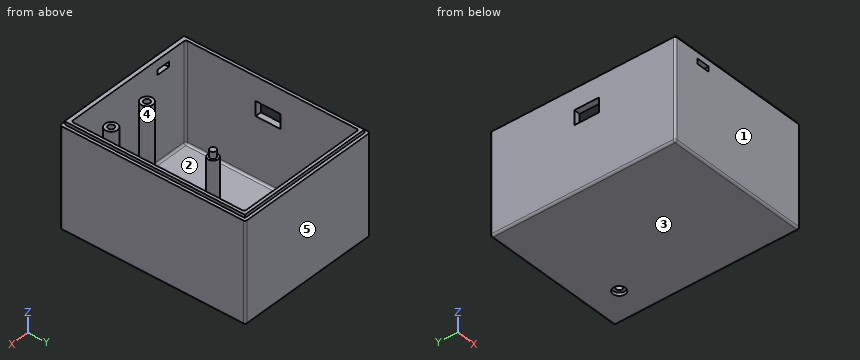
```python
from build123d import *

# Parameters (mm, degrees)
SKETCH1_W                    = 71
SKETCH1_H                    = 90
BOSS_EXTRUDE1_DEPTH          = 50
SHELL1_T                     = -3
SHELL1_THICKNESS_2_FACE_W    = 65
SHELL1_THICKNESS_2_FACE_H    = 84
SHELL1_THICKNESS_2_DEPTH     = 1
SKETCH3_W                    = 6.5
SKETCH3_H                    = 2.5
CUT_EXTRUDE1_DEPTH           = 3
SKETCH4_W                    = 7
SKETCH4_H                    = 12
CUT_EXTRUDE2_DEPTH           = 3
SKETCH5_R                    = 3
SKETCH5_R_2                  = 2.5
BOSS_EXTRUDE2_DEPTH          = 38
F_3_0_3_DIAMETER_HOLE1_D     = 3
F_3_0_3_DIAMETER_HOLE1_DEPTH = 8.5
F_3_0_3_DIAMETER_HOLE1_TIP   = 0.901290929
FILLET1_R                    = 1
FILLET2_R                    = 1
SKETCH22_R                   = 1.5
BOSS_EXTRUDE4_DEPTH          = 3.3
SKETCH23_R                   = 3
BOSS_EXTRUDE5_DEPTH          = 4
CUT_EXTRUDE3_START           = -1.5
CUT_EXTRUDE3_DEPTH           = 1.5
CUT_EXTRUDE4_DEPTH           = 68
SKETCH29_R                   = 3
CUT_EXTRUDE5_DEPTH           = 1.5
SKETCH30_R                   = 1.5
CUT_EXTRUDE6_DEPTH           = 2.5


# Read off the part's stored shape, not the designer's step: Cut-Extrude3
with BuildPart() as part:
    # Sketch1 → Boss-Extrude1 (new body)
    with BuildSketch(Plane.XY):
        Rectangle(SKETCH1_W, SKETCH1_H)
    extrude(amount=-BOSS_EXTRUDE1_DEPTH)

    # Shell1
    shell1_openings = [part.faces().sort_by_distance(p)[0] for p in [
        (0, 0, 0),
    ]]
    offset(amount=SHELL1_T, openings=shell1_openings, kind=Kind.INTERSECTION)

    # Shell1 thickness 2 face (on inner face of the shell) → Shell1 thickness 2 (cut)
    with BuildSketch(Plane(origin=(0, 0, -47), x_dir=(-1, 0, 0), z_dir=(0, 0, -1))):
        Rectangle(SHELL1_THICKNESS_2_FACE_W, SHELL1_THICKNESS_2_FACE_H)
    extrude(amount=SHELL1_THICKNESS_2_DEPTH, mode=Mode.SUBTRACT)

    # Sketch3 → Cut-Extrude1 (cut)
    with BuildSketch(Plane.XZ.offset(45)):
        with Locations((-19.75, -5.75)):
            Rectangle(SKETCH3_W, SKETCH3_H)
    extrude(amount=-CUT_EXTRUDE1_DEPTH, mode=Mode.SUBTRACT)

    # Sketch4 → Cut-Extrude2 (cut)
    with BuildSketch(Plane.ZY.offset(35.5)):
        with Locations((-15, -2)):
            Rectangle(SKETCH4_W, SKETCH4_H)
    extrude(amount=-CUT_EXTRUDE2_DEPTH, mode=Mode.SUBTRACT)

    # Sketch5 → Boss-Extrude2 (add)
    with BuildSketch(Plane.XY.offset(-48)):
        with Locations((-4.82, -37.13)):
            Circle(SKETCH5_R)
        with Locations((15.5, -37.13)):
            Circle(SKETCH5_R)
        with Locations((4.83, 3.15)):
            Circle(SKETCH5_R_2)
    extrude(amount=BOSS_EXTRUDE2_DEPTH)

    # Ø3.0 (3) Diameter Hole1
    with Locations(Plane.XY.offset(-10)):
        with Locations((-4.82, -37.13), (15.5, -37.13), (15.5, 6.05), (-4.82, 6.05)):
            Hole(F_3_0_3_DIAMETER_HOLE1_D / 2, depth=F_3_0_3_DIAMETER_HOLE1_DEPTH)
            with Locations((0, 0, -(F_3_0_3_DIAMETER_HOLE1_DEPTH + F_3_0_3_DIAMETER_HOLE1_TIP / 2))):  # 118° drill point
                Cone(0, F_3_0_3_DIAMETER_HOLE1_D / 2, F_3_0_3_DIAMETER_HOLE1_TIP, mode=Mode.SUBTRACT)

    # Fillet1
    fillet1_edges = [part.edges().sort_by_distance(p)[0] for p in [
        (-35.5, 0, -50),
        (0, -45, -50),
        (32.5, 42, -24),
        (32.5, -42, -24),
        (-32.5, -42, -24),
        (-32.5, 42, -24),
        (35.5, 0, -50),
        (0, 45, -50),
        (35.5, -45, -25),
        (-35.5, -45, -25),
        (-35.5, 45, -25),
        (35.5, 45, -25),
    ]]
    fillet(fillet1_edges, radius=FILLET1_R)

    # Fillet2
    # the kernel refuses this fillet: 1 mm, written as the material it adds along each edge
    with BuildSketch(Plane(origin=(-4.82, -37.13, -48), x_dir=(1, 0, 0), z_dir=(0, -1, 0))) as fillet2_piece_1:
        with BuildLine():
            CenterArc((3 + FILLET2_R, FILLET2_R), FILLET2_R, 180, 90)
            Line((3, FILLET2_R), (3, 0))
            Line((3, 0), (3 + FILLET2_R, 0))
        make_face()
    revolve(axis=Axis((-4.82, -37.13, -48), (0, 0, 1)))
    with BuildSketch(Plane(origin=(15.5, -37.13, -48), x_dir=(1, 0, 0), z_dir=(0, -1, 0))) as fillet2_piece_2:
        with BuildLine():
            CenterArc((3 + FILLET2_R, FILLET2_R), FILLET2_R, 180, 90)
            Line((3, FILLET2_R), (3, 0))
            Line((3, 0), (3 + FILLET2_R, 0))
        make_face()
    revolve(axis=Axis((15.5, -37.13, -48), (0, 0, 1)))
    with BuildSketch(Plane(origin=(4.83, 3.15, -48), x_dir=(1, 0, 0), z_dir=(0, -1, 0))) as fillet2_piece_3:
        with BuildLine():
            CenterArc((2.5 + FILLET2_R, FILLET2_R), FILLET2_R, 180, 90)
            Line((2.5, FILLET2_R), (2.5, 0))
            Line((2.5, 0), (2.5 + FILLET2_R, 0))
        make_face()
    revolve(axis=Axis((4.83, 3.15, -48), (0, 0, 1)))
    with BuildSketch(Plane(origin=(31.5, 42, -48), x_dir=(0, 0, 1), z_dir=(-1, 0, 0)), Plane(origin=(-31.5, -42, -48), x_dir=(0, 0, 1), z_dir=(1, 0, 0))) as fillet2_piece_4:
        with BuildLine():
            CenterArc((FILLET2_R, -FILLET2_R), FILLET2_R, 90, 90)
            Line((0, -FILLET2_R), (0, 0))
            Line((0, 0), (FILLET2_R, 0))
        make_face()
    extrude(amount=63)
    with BuildSketch(Plane(origin=(32.5, -41, -48), x_dir=(0, 0, 1), z_dir=(0, 1, 0)), Plane(origin=(-32.5, 41, -48), x_dir=(0, 0, 1), z_dir=(0, -1, 0))) as fillet2_piece_5:
        with BuildLine():
            CenterArc((FILLET2_R, -FILLET2_R), FILLET2_R, 90, 90)
            Line((0, -FILLET2_R), (0, 0))
            Line((0, 0), (FILLET2_R, 0))
        make_face()
    extrude(amount=82)
    with BuildSketch(Plane(origin=(-31.5, -41, -48), x_dir=(-1, 0, 0), z_dir=(0, 1, 0))) as fillet2_piece_6:
        with BuildLine():
            CenterArc((1 - FILLET2_R, FILLET2_R), FILLET2_R, 270, 90)
            Line((1 - FILLET2_R, 0), (1, 0))
            Line((1, 0), (1, FILLET2_R))
        make_face()
    revolve(axis=Axis((-31.5, -41, -48), (0, 0, 1)), revolution_arc=90)
    with BuildSketch(Plane(origin=(-31.5, 41, -48), x_dir=(0, 1, 0), z_dir=(1, 0, 0))) as fillet2_piece_7:
        with BuildLine():
            CenterArc((1 - FILLET2_R, FILLET2_R), FILLET2_R, 270, 90)
            Line((1 - FILLET2_R, 0), (1, 0))
            Line((1, 0), (1, FILLET2_R))
        make_face()
    revolve(axis=Axis((-31.5, 41, -48), (0, 0, 1)), revolution_arc=90)
    with BuildSketch(Plane(origin=(31.5, -41, -48), x_dir=(0, -1, 0), z_dir=(-1, 0, 0))) as fillet2_piece_8:
        with BuildLine():
            CenterArc((1 - FILLET2_R, FILLET2_R), FILLET2_R, 270, 90)
            Line((1 - FILLET2_R, 0), (1, 0))
            Line((1, 0), (1, FILLET2_R))
        make_face()
    revolve(axis=Axis((31.5, -41, -48), (0, 0, 1)), revolution_arc=90)
    with BuildSketch(Plane(origin=(31.5, 41, -48), x_dir=(0, 1, 0), z_dir=(-1, 0, 0))) as fillet2_piece_9:
        with BuildLine():
            CenterArc((1 - FILLET2_R, -FILLET2_R), FILLET2_R, 0, 90)
            Line((1 - FILLET2_R, 0), (1, 0))
            Line((1, 0), (1, -FILLET2_R))
        make_face()
    revolve(axis=Axis((31.5, 41, -48), (0, 0, -1)), revolution_arc=90)

    # Sketch22 → Boss-Extrude4 (add)
    with BuildSketch(Plane.XY.offset(-10)):
        with Locations((4.83, 3.15)):
            Circle(SKETCH22_R)
    extrude(amount=BOSS_EXTRUDE4_DEPTH)

    # Sketch23 → Boss-Extrude5 (add)
    with BuildSketch(Plane(origin=(0, 0, -50), x_dir=(-1, 0, 0), z_dir=(0, 0, -1))):
        with Locations((-20.5, 30)):
            Circle(SKETCH23_R)
    extrude(amount=-BOSS_EXTRUDE5_DEPTH)

    # Cut-Extrude3 outline → Cut-Extrude3 (cut)
    with BuildSketch(Plane.XY.offset(CUT_EXTRUDE3_START)):
        with BuildLine():
            Line((-34, 43.5), (34, 43.5))
            Line((34, 43.5), (34, -45))
            Line((34, -45), (34.5, -45))
            ThreePointArc((34.5, -45), (35.207106781, -44.707106781), (35.5, -44))
            Line((35.5, -44), (35.5, 44))
            ThreePointArc((35.5, 44), (35.207106781, 44.707106781), (34.5, 45))
            Line((34.5, 45), (-34.5, 45))
            ThreePointArc((-34.5, 45), (-35.207106781, 44.707106781), (-35.5, 44))
            Line((-35.5, 44), (-35.5, -44))
            ThreePointArc((-35.5, -44), (-35.207106781, -44.707106781), (-34.5, -45))
            Line((-34.5, -45), (-34, -45))
            Line((-34, -45), (-34, 43.5))
        make_face()
    extrude(amount=CUT_EXTRUDE3_DEPTH, mode=Mode.SUBTRACT)

    # Sketch26 → Cut-Extrude4 (cut)
    with BuildSketch(Plane.ZY.offset(34)):
        Polygon((0, -45), (0, -44), (-1.5, -43.5), (-1.5, -45), align=None)
    extrude(amount=-CUT_EXTRUDE4_DEPTH, mode=Mode.SUBTRACT)

    # Sketch29 → Cut-Extrude5 (cut)
    with BuildSketch(Plane(origin=(0, 0, -50), x_dir=(-1, 0, 0), z_dir=(0, 0, -1))):
        with Locations((-20.5, 30)):
            Circle(SKETCH29_R)
    extrude(amount=-CUT_EXTRUDE5_DEPTH, mode=Mode.SUBTRACT)

    # Sketch30 → Cut-Extrude6 (cut)
    with BuildSketch(Plane(origin=(0, 0, -48.5), x_dir=(-1, 0, 0), z_dir=(0, 0, -1))):
        with Locations((-20.5, 30)):
            Circle(SKETCH30_R)
    extrude(amount=-CUT_EXTRUDE6_DEPTH, mode=Mode.SUBTRACT)


solid = part.part
```
Verification items for the finished model (mm, model axes). Face numbers are marked on the shaded views. A direction names the side the tool comes from. Give positions to 0.01 mm unless a question says otherwise; leave off trailing zeros. Loops run counter-clockwise (first coordinate to the right, second up) from the corner with the lowest first, then second, coordinate; pieces in that order, holes last. Notation, with made-up numbers: M -3.5,84 L 47.5,84 A25 cw 47.5,105 Z; hole C -15.75,39.25 d7. An arc over 180 degrees is marked long. Return JSON: item names as keys, results as strings.
1) Section check D-D, the plane y = -4. Enter the section's corners in (x, z), and give its area (4 significant figures).
Findings:
{"outline": "M -35.5,-49 A1 ccw -34.5,-50 L 34.5,-50 A1 ccw 35.5,-49 L 35.5,-1.5 L 34,-1.5 L 34,0 L 32.5,0 L 32.5,-47 A1 cw 31.5,-48 L -31.5,-48 A1 cw -32.5,-47 L -32.5,-18.5 L -35.5,-18.5 Z; M -35.5,-11.5 L -32.5,-11.5 L -32.5,0 L -34,0 L -34,-1.5 L -35.5,-1.5 Z", "area": "404.5 mm2"}
2) Section check B-B, the plane z = -27. Enter the section's corners in (x, y), and give its area (3 significant figures).
Findings:
{"outline": "M -35.5,-44 A1 ccw -34.5,-45 L 34.5,-45 A1 ccw 35.5,-44 L 35.5,44 A1 ccw 34.5,45 L -34.5,45 A1 ccw -35.5,44 Z; C -4.82,-37.13 d6; C 4.83,3.15 d5; C 15.5,-37.13 d6; hole M -32.5,-41 A1 ccw -31.5,-42 L 31.5,-42 A1 ccw 32.5,-41 L 32.5,41 A1 ccw 31.5,42 L -31.5,42 A1 ccw -32.5,41 Z", "area": "1,010 mm2"}
3) Tool access check on the marked faces 4 and 5. Record the directions out of +Z, -Z, +X, -X, +Y, -Y that give a thin tool (end or side, any length) a straight path to the whole face; none if there is none.
Findings:
{"face 4": "+Z", "face 5": "+Z, -Z, +X, -X, +Y"}
4) Mould release check, pull along Y, two halves, no side actions. Record for the marked faces 1, 2 and 3: released by +Y, released by -Y, zero draft, split by the parting line, or undercut.
Findings:
{"face 1": "released by -Y", "face 2": "undercut", "face 3": "zero draft"}
5) Section check A-A, the plane y = 30. Enter the section's corners in (x, z), and give its area (3 significant figures).
Findings:
{"outline": "M -35.5,-49 A1 ccw -34.5,-50 L 17.5,-50 L 17.5,-48.5 L 19,-48.5 L 19,-46 L 17.5,-46 L 17.5,-48 L -31.5,-48 A1 cw -32.5,-47 L -32.5,0 L -34,0 L -34,-1.5 L -35.5,-1.5 Z; M 22,-48.5 L 23.5,-48.5 L 23.5,-50 L 34.5,-50 A1 ccw 35.5,-49 L 35.5,-1.5 L 34,-1.5 L 34,0 L 32.5,0 L 32.5,-47 A1 cw 31.5,-48 L 23.5,-48 L 23.5,-46 L 22,-46 Z", "area": "421 mm2"}
6) Section check C-C, the plane x = 4.83. Enter the section's corners in (y, z), and give its area (3 significant figures).
Findings:
{"outline": "M -45,-49 A1 ccw -44,-50 L 44,-50 A1 ccw 45,-49 L 45,-1.5 L 43.5,-1.5 L 43.5,0 L 42,0 L 42,-47 A1 cw 41,-48 L 6.65,-48 A1 cw 5.65,-47 L 5.65,-10 L 4.65,-10 L 4.65,-6.7 L 1.65,-6.7 L 1.65,-10 L 0.65,-10 L 0.65,-47 A1 cw -0.35,-48 L -41,-48 A1 cw -42,-47 L -42,0 L -44,0 L -43.5,-1.5 L -45,-1.5 Z", "area": "664 mm2"}
7) Material ranges on L1, parallel to Y at x = 5, z = -24.5; L2, parallel to Y at x = -4.82, z = -13.75; L3, parallel to Y at x = -29, z = -35.5, recorded low to high. Write a range as [from, to].
Findings:
{"L1": "y = [-45, -42], [0.66, 5.64], [42, 45]", "L2": "y = [-45, -42], [-40.13, -38.63], [-35.63, -34.13], [42, 45]", "L3": "y = [-45, -42], [42, 45]"}
8) Gauge pin test, flat ends, axial feed: P1, Ø1.5, axis at x = 25, y = 22, coming from the +Z side; P2, Ø0.8, axis at y = 9.5, z = -0.5, coming from the +X side; P3, Ø1.8, axis at x = 19, y = 31, coming from the +Z side. Record the tip position at first contact, or that the pin passes through.
Findings:
{"P1": "stops at z = -48", "P2": "stops at x = 34", "P3": "stops at z = -46"}
